```python
from build123d import *

# Parameters (mm, degrees)
F1_DEPTH = 2
F4_COUNT = 6
F4_ANGLE = 300


with BuildPart() as f1:
    # F0 (on Top) → F1 (new body)
    with BuildSketch(Plane.XY):
        Polygon((0, 95), (0, 0), (9.0951109305, 0), (15.0057672536, 11.6038580467), (5.1223551854, 16.6381709278), (9.968268685, 33.868085593), (21.4383043349, 48.3848489821), (6.0254437849, 55.9120550752), (26.4652259648, 69.2315325141), (38.8642698526, 65.456263721), (42.6333136857, 69.7637423873), (27.5425929576, 78.0722051859), (6.3733253418, 70.0200916975), (3.6955948453, 77.0599320531), (11.7607787251, 78.0722051859), (20.7214262336, 84.4079181552), (12.1189001948, 91.5766954422), align=None)
    extrude(amount=F1_DEPTH)

    # F2: F1 across plane


with BuildPart() as f1_1:
    add(f1.part)
    add(f1.part.mirror(Plane.YZ))

    # F4: F1 ×6 about axis
    f4_axis = Axis((0, 0, 4.1130185127), (0, 0, 1))


with BuildPart() as f1_2:
    add(f1_1.part)
    for i in range(1, F4_COUNT):
        add(f1_1.part.rotate(f4_axis, i * F4_ANGLE / (F4_COUNT - 1)))


solid = f1_2.part
```
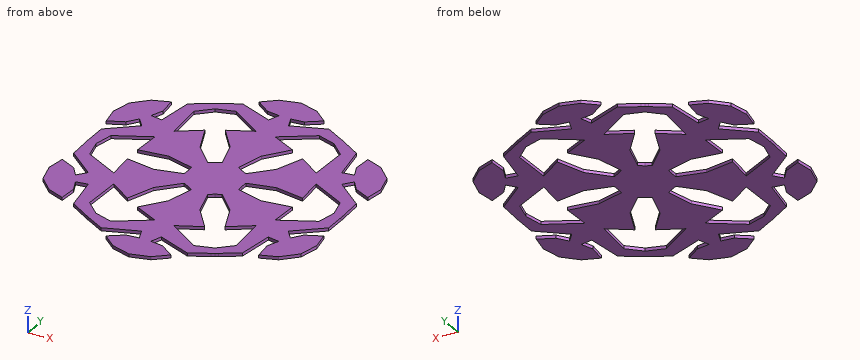
Input: part model. Units: mm. Frame: model coordinates. Coordinates: 2 decimals unless noted, no trailing zeros. Order: outer loops, then holes, each group sorted by start corner. A loop starts at its lowest first (then second) coordinate and runs counter-clockwise, first axis right, second up. Notation, with made-up numbers: (-15.5, 86.5) - (-11.5, 86.5) arc R9 cw to (-11.5, 92.5) - close; hole circle Ø3 at (75, 73). An arc over 180 degrees is marked (long way). Return JSON: item names as keys, results as strings.
Q1. Cut plane B-B (z = 1.5). State how many separate pieces and enclosed holes the cut face has, then the cut area to 3 significant figures.
The answers:
{"separate pieces": "1", "enclosed holes": "6", "area": "14,900 mm2"}
Q2. First-contact query: pin 1 (1 mm diameter, centred on x = -4.5, z = 0.5, fed in from -Y). Flat tip, straight axial feed; report the tip coordinate or a pass-through.
The answers:
{"pin 1": "stops at y = -93.87"}
Q3. Cut plane A-A (x = -15). Return loops of the section in (y, z), then the cut area to 3 significant figures.
The answers:
{"outline": "(-89.18, 0) - (-80.36, 0) - (-80.36, 2) - (-89.18, 2) - close; (-73.3, 0) - (-61.76, 0) - (-61.76, 2) - (-73.3, 2) - close; (-51.53, 0) - (-40.24, 0) - (-40.24, 2) - (-51.53, 2) - close; (-15.99, 0) - (15.99, 0) - (15.99, 2) - (-15.99, 2) - close; (40.24, 0) - (51.53, 0) - (51.53, 2) - (40.24, 2) - close; (61.76, 0) - (73.3, 0) - (73.3, 2) - (61.76, 2) - close; (80.36, 0) - (89.18, 0) - (89.18, 2) - (80.36, 2) - close", "area": "191 mm2"}
Q4. Ray query, probe 1 along Y at (x, z) = (41, 1.3); probe 2 along X at (y, z) = (-23.5, 1.8); probe 3 along Y at (x, z) = (67, 1). Return the intervals inside material, ascending.
The answers:
{"probe 1": "y = -70.66 to -62.88, -36.14 to -7.32, 7.32 to 36.14, 62.88 to 70.66", "probe 2": "x = -71.18 to -22.33, -7.05 to 7.05, 22.33 to 71.18", "probe 3": "y = -58.58 to -33.39, -26.9 to -14.84, 14.84 to 26.9, 33.39 to 58.58"}
